```python
from build123d import *

# Parameters (mm, degrees)
F1_DEPTH = 254
F2_R     = 25.4
F4_DEPTH = 25.4
F5_R     = 12.7
F6_R     = 25.4
F7_DEPTH = 25.4


with BuildPart() as f1:
    # F0 (on Front) → F1 (new body)
    with BuildSketch(Plane.XZ):
        with BuildLine():
            Line((-558.8, -63.5), (0, -63.5))
            ThreePointArc((0, -63.5), (44.9012806053, -44.9012806053), (63.5, 0))
            Line((63.5, 0), (63.5, 330.2))
            Line((63.5, 330.2), (38.1, 330.2))
            Line((38.1, 330.2), (38.1, 0))
            ThreePointArc((38.1, 0), (26.9407683632, -26.9407683632), (0, -38.1))
            Line((0, -38.1), (-558.8, -38.1))
            Line((-558.8, -38.1), (-558.8, -63.5))
        make_face()
    extrude(amount=F1_DEPTH)

    # F2
    f2_edges = [f1.edges().sort_by_distance(p)[0] for p in [
        (50.8, 0, 330.2),
        (50.8, -254, 330.2),
        (-558.8, 0, -50.8),
        (-558.8, -254, -50.8),
    ]]
    fillet(f2_edges, radius=F2_R)

    # F3 (on face) → F4 (cut)
    with BuildSketch(Plane.XY.offset(-38.1)):
        with BuildLine():
            Line((-348.8516446213, -101.6), (-484.7166538239, -101.6))
            Line((-484.7166538239, -101.6), (-484.7166538239, -152.4))
            Line((-484.7166538239, -152.4), (-348.8516446213, -152.4))
            ThreePointArc((-348.8516446213, -152.4), (-354.4673153923, -127), (-348.8516446213, -101.6))
        make_face()
        with BuildLine():
            ThreePointArc((-239.5816630264, -101.6), (-294.2166538239, -66.7493384316), (-348.8516446213, -101.6))
            Line((-348.8516446213, -101.6), (-239.5816630264, -101.6))
        make_face()
        with BuildLine():
            Line((-239.5816630264, -101.6), (-348.8516446213, -101.6))
            ThreePointArc((-348.8516446213, -101.6), (-354.4673153923, -127), (-348.8516446213, -152.4))
            Line((-348.8516446213, -152.4), (-239.5816630264, -152.4))
            ThreePointArc((-239.5816630264, -152.4), (-235.3866590943, -140.0066882623), (-233.9659922554, -127))
            ThreePointArc((-233.9659922554, -127), (-235.3866590943, -113.9933117377), (-239.5816630264, -101.6))
        make_face()
        with BuildLine():
            Line((-103.7166538239, -101.6), (-239.5816630264, -101.6))
            ThreePointArc((-239.5816630264, -101.6), (-235.3866590943, -113.9933117377), (-233.9659922554, -127))
            ThreePointArc((-233.9659922554, -127), (-235.3866590943, -140.0066882623), (-239.5816630264, -152.4))
            Line((-239.5816630264, -152.4), (-103.7166538239, -152.4))
            Line((-103.7166538239, -152.4), (-103.7166538239, -101.6))
        make_face()
        with BuildLine():
            Line((-239.5816630264, -152.4), (-348.8516446213, -152.4))
            ThreePointArc((-348.8516446213, -152.4), (-294.2166538239, -187.2506615684), (-239.5816630264, -152.4))
        make_face()
    extrude(amount=-F4_DEPTH, mode=Mode.SUBTRACT)

    # F5
    f5_edges = [f1.edges().sort_by_distance(p)[0] for p in [
        (-484.716654, -101.6, -50.8),
        (-348.851645, -101.6, -50.8),
        (-484.716654, -152.4, -50.8),
        (-348.851645, -152.4, -50.8),
        (-239.581663, -152.4, -50.8),
        (-239.581663, -101.6, -50.8),
        (-103.716654, -152.4, -50.8),
        (-103.716654, -101.6, -50.8),
    ]]
    fillet(f5_edges, radius=F5_R)

    # F6 (on face) → F7 (cut)
    with BuildSketch(Plane.YZ.offset(63.5)):
        with Locations((-50.8, 279.4)):
            Circle(F6_R)
        with Locations((-203.2, 279.4)):
            Circle(F6_R)
        with Locations((-50.8, 97.3987299839)):
            Circle(F6_R)
        with Locations((-203.2, 97.3987299839)):
            Circle(F6_R)
    extrude(amount=-F7_DEPTH, mode=Mode.SUBTRACT)


solid = f1.part
```
Geometry: final body of the model. Coordinates: model frame, mm. A direction names the side the tool comes from. Round coordinates to 2 decimals unless told otherwise and drop trailing zeros. Write each loop counter-clockwise with the first axis right and the second up, starting at its lowest first coordinate (ties: lowest second). Pieces come first, ordered by that corner, then holes. Notation, with made-up numbers: M 85.5,-18.5 L 122.5,-18.5 A20 ccw 122.5,-2.5 Z; hole C 28.5,-27 d5. An arc over 180 degrees is marked long. Answer in a Markdown table with one row per item. Add a question column.
(1) Cut plane D-D, the plane y = -166. Return the cut outline in (x, z), then the cut area to 3 significant figures.
(2) Cut plane C-C, the plane y = -50.8. Return the cut outline in (x, z), then the cut area to 3 significant figures.
(3) Contact query for flat-ended pins moving along their axis: pin 1 (5 mm diameter, centred on y = -116, z = 204.5, fed in from -X); pin 2 (6 mm diameter, centred on x = -30.5, y = -166.5, fed in from +Z); pin 3 (20.5 mm diameter, centred on y = -128.5, z = -50.5, fed in from +X). Output: stop coordinate, or through.
(4) Cut plane B-B, the plane x = -413.5. Return the cut outline in (y, z), then the cut area to 3 significant figures.
(5) Draft query along Z for faces 4 (the face through (50.978, -179.737, 87.67)), 5 (the face through (51, -126, 330.2)), 6 (the face through (-148, -254, -42)). Return one class per face: pulls with the +Z half, pulls with the -Z half, needs draft (parallel to the pull), parting line crosses it, or undercut.
(6) Cut plane A-A, the plane z = 279.4. Return the cut outline in (x, y).
(7) Ray query, L1, parallel to Y at x = 56, z = 279; L2, parallel to Z at x = 58.25, y = -203.2; L3, parallel to Z at x = 58, y = -50.8. Return the intervals inside material, ascending.
(8) Reachability of faces 1 (the face through (-413, -101.6, -51)), 2 (the face through (-275, -69, -38.1)), 3 (the face through (50.98, -189.55, 300.82)) from +Z, -Z, +X, -X, +Y, -Y: full face, straight path, thin tool, end or side. Return the list, or none.
Established:
| question | item | result |
|---|---|---|
| 1 | outline | M -558.8,-63.5 L -340.14,-63.5 L -340.14,-38.1 L -558.8,-38.1 Z; M -248.29,-63.5 L 0,-63.5 A63.5 ccw 63.5,0 L 63.5,330.2 L 38.1,330.2 L 38.1,0 A38.1 cw 0,-38.1 L -248.29,-38.1 Z |
| 1 | area | 22,300 mm² |
| 2 | outline | M -558.8,-63.5 L 0,-63.5 A63.5 ccw 63.5,0 L 63.5,72 L 38.1,72 L 38.1,0 A38.1 cw 0,-38.1 L -558.8,-38.1 Z; M 38.1,122.8 L 63.5,122.8 L 63.5,254 L 38.1,254 Z; M 38.1,304.8 L 63.5,304.8 L 63.5,330.2 L 38.1,330.2 Z |
| 2 | area | 22,000 mm² |
| 3 | pin 1 | x = 38.1 |
| 3 | pin 2 | z = -38.1 |
| 3 | pin 3 | x = 49.11 |
| 4 | outline | M -254,-63.5 L -152.4,-63.5 L -152.4,-38.1 L -254,-38.1 Z; M -101.6,-63.5 L 0,-63.5 L 0,-38.1 L -101.6,-38.1 Z |
| 4 | area | 5,160 mm² |
| 5 | face 4 | undercut |
| 5 | face 5 | pulls with the +Z half |
| 5 | face 6 | needs draft |
| 6 | outline | M 38.1,-254 L 63.5,-254 L 63.5,-228.6 L 38.1,-228.6 Z; M 38.1,-177.8 L 63.5,-177.8 L 63.5,-76.2 L 38.1,-76.2 Z; M 38.1,-25.4 L 63.5,-25.4 L 63.5,0 L 38.1,0 Z |
| 7 | L1 | -254 to -228.6, -177.8 to -76.2, -25.4 to 0 |
| 7 | L2 | -25.28 to 72, 122.8 to 254, 304.8 to 330.2 |
| 7 | L3 | -25.85 to 72, 122.8 to 254, 304.8 to 330.2 |
| 8 | face 1 | +Z, -Z |
| 8 | face 2 | +Z, -X, +Y, -Y |
| 8 | face 3 | +X, -X |
